The listing builds one solid part. Answer for the finished solid, in the listing's coordinates (mm). Face numbers are marked on the shaded views. Coordinates: 2 decimals unless noted, no trailing zeros. Order: outer loops, then holes, each group sorted by start corner. A loop starts at its lowest first (then second) coordinate and runs counter-clockwise, first axis right, second up. Notation, with made-up numbers: (-17.5, -5.75) -> (-13.5, -5.75) arc R30 cw to (-13.5, 18.25) -> close; hole circle Ø10 at (-4, 47.25). An arc over 180 degrees is marked (long way). One line per question, with ' | ' between items.
from build123d import *

# Parameters (mm, degrees)
EXTRUDE_1_DEPTH     = 50
SKETCH_2_R          = 2.15
CUT_EXTRUDE_1_DEPTH = 18


with BuildPart() as part:
    # 草图1 → 凸台-拉伸1 (new body)
    with BuildSketch(Plane(origin=(0, 0, 0), x_dir=(0, 0, -1), z_dir=(1, 0, 0))):
        Polygon((117.696324268, -1.952846431), (117.696324268, -11.952846431), (-32.303675732, -11.952846431), (-2.303675732, 40.008677796), (6.356578306, 35.008677796), (-14.983167656, -1.952846431), align=None)
    extrude(amount=EXTRUDE_1_DEPTH)

    # 草图2 → 切除-拉伸1 (cut)
    with BuildSketch(Plane(origin=(0, 10.999690302, 19.052022471), x_dir=(1, 0, 0), z_dir=(0, 0.5, 0.866025404))):
        with Locations((25, -1.503306522)):
            Circle(SKETCH_2_R)
    extrude(amount=-CUT_EXTRUDE_1_DEPTH, mode=Mode.SUBTRACT)


solid = part.part
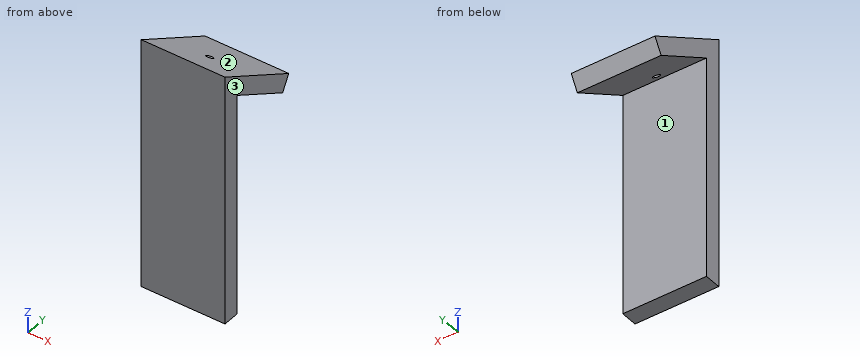
Item 1: Find the intervals of material crossed by L1, parallel to Y at x = 36.5, z = -76.5; L2, parallel to Y at x = 14.5, z = 7.5; L3, parallel to Y at x = 15.5, z = -3, in increasing order.
Computed values:
L1: y = -11.95 to -1.95 | L2: y = -11.95 to -1.95, 11.01 to 31.01 | L3: y = -11.95 to -1.95, 29.19 to 36.95
Item 2: Section D-D, the plane y = 0.5 is taken. Give the vertices of the cut face in (x, z), plus the area to 3 significant figures.
Computed values:
outline: (0, 13.57) -> (50, 13.57) -> (50, 25.11) -> (0, 25.11) -> close | area: 577 mm^2
Item 3: Determine the mould class of the marked faces 1, 2 and 3 for opening direction Y: pulls with the +Y half, pulls with the -Y half, needs draft (parallel to the pull), parting line crosses it, or undercut.
Computed values:
face 1: undercut | face 2: pulls with the +Y half | face 3: needs draft
Item 4: Each of these flat-tipped pins is pushed along its axis until it touches: pin 1 Ø25 at (x, z) = (14.5, -18.5) entering from +Y; pin 2 Ø12 at (x, y) = (16.5, 12.5) entering from -Z; pin 3 Ø5 at (x, y) = (20, 19.5) entering from -Z; pin 4 Ø5 at (y, z) = (10.5, 6.5) entering from +X. Where does it stop, or does it pass through?
Computed values:
pin 1: stops at y = 35.21 | pin 2: stops at z = 3.17 | pin 3: stops at z = 1.15 | pin 4: stops at x = 50
Item 5: Section A-A, the plane x = 42 is taken. Give the vertices of the cut face in (y, z).
Computed values:
outline: (-11.95, -117.7) -> (-1.95, -117.7) -> (-1.95, 14.98) -> (35.01, -6.36) -> (40.01, 2.3) -> (-11.95, 32.3) -> close
Item 6: Section B-B, the plane z = 6 is taken. Give the vertices of the cut face in (x, y), plus the area to 3 significant figures.
Computed values:
outline: (0, -11.95) -> (50, -11.95) -> (50, -1.95) -> (0, -1.95) -> close; (0, 13.61) -> (50, 13.61) -> (50, 33.61) -> (0, 33.61) -> close | area: 1,500 mm^2
Item 7: Section C-C, the plane z = -78 is taken. Give the vertices of the cut face in (x, y), plus the area to 3 significant figures.
Computed values:
outline: (0, -11.95) -> (50, -11.95) -> (50, -1.95) -> (0, -1.95) -> close | area: 500 mm^2
